```python
from build123d import *

# Parameters (mm, degrees)
F0_W     = 10
F0_H     = 10
F1_DEPTH = 10
F2_W     = 5
F2_H     = 5
F3_DEPTH = 5
F4_W     = 5
F4_H     = 5
F5_DEPTH = 5
F6_W     = 5
F6_H     = 5
F7_DEPTH = 5
F8_R     = 1.295802
F9_DEPTH = 25


with BuildPart() as f1:
    # F0 (on Top) → F1 (new body)
    with BuildSketch(Plane.XY):
        with Locations((-5, 5)):
            Rectangle(F0_W, F0_H)
    extrude(amount=F1_DEPTH)

    # F2 (on face) → F3 (join)
    with BuildSketch(Plane.YZ):
        with Locations((7.5, 2.5)):
            Rectangle(F2_W, F2_H)
    extrude(amount=F3_DEPTH)

    # F4 (on face) → F5 (join)
    with BuildSketch(Plane.XZ):
        with Locations((-7.5, 2.5)):
            Rectangle(F4_W, F4_H)
    extrude(amount=F5_DEPTH)

    # F6 (on face) → F7 (join)
    with BuildSketch(Plane.XY.offset(10)):
        with Locations((-7.5, 7.5)):
            Rectangle(F6_W, F6_H)
    extrude(amount=F7_DEPTH)

    # F8 (on face) → F9 (cut)
    with BuildSketch(Plane.XY.offset(15)):
        with Locations((-7.5, 7.526434)):
            Circle(F8_R)
    extrude(amount=-F9_DEPTH, mode=Mode.SUBTRACT)


solid = f1.part
```
Could you check a few things on this model? Use its own coordinates, in mm. A direction names the side the tool comes from. Round coordinates to 2 decimals unless told otherwise and drop trailing zeros. Loops run counter-clockwise (first coordinate to the right, second up) from the corner with the lowest first, then second, coordinate; pieces in that order, holes last. Notation, with made-up numbers: (7.5, 86) - (54.5, 86) arc R16 cw to (54.5, 97) - close; hole circle Ø11 at (36, -34.75). An arc over 180 degrees is marked (long way). Answer in a Markdown table with one row per item. Add a question column.
(1) If we section it at B-B (y = 8.5): Please give me the cut outline in (x, z), plus the area to 3 significant figures.
(2) I'm going to push flat-ended pins straight in: pin 1 (5.5 mm diameter, centred on x = 2, z = 2, fed in from -Y); pin 2 (4 mm diameter, centred on x = 3.5, y = 7.5, fed in from +Z); pin 3 (1.5 mm diameter, centred on x = -4, y = -2.5, fed in from -Z); pin 4 (2 mm diameter, centred on y = 1.5, z = 6, fed in from +X). Where does each tip first touch, or does it pass through?
(3) If we mould it in two halves opening along X, with no side actions, what happens to faces 1 (the face through (-10, 4, 6)), 2 (the face through (5, 7, 3)), 3 (the face through (-6.803, 8.619, 7.605)), 4 (the face through (-8, -2, 5))? For each: pulls with the +X half, pulls with the -X half, needs draft (parallel to the pull), parting line crosses it, or undercut.
(4) If we section it at D-D (x = -5.75): Please give me the cut outline in (y, z).
(5) I need wall thicknesses on line 1 along Y through (x, z) = (-7.5, 6.5); line 2 along X through (y, z) = (-2.25, 2.5); line 3 along X through (y, z) = (2.5, 4.5). Which ranges of each line are inside material? Lowest first, please.
(6) If we section it at A-A (x = -7.5): Please give me the cut outline in (y, z), plus the area to 3 significant figures.
(7) For faces 5 (the face through (-8, 5, 12)), 6 (the face through (2, 7, 5)), 7 (the face through (-8, -5, 3)), 8 (the face through (-5, -2, 2)), 9 (the face through (-4, 4, 0)), which set-ups out of +Z, -Z, +X, -X, +Y, -Y let a thin tool reach every point of the face, with its end or its side?
(8) If we section it at C-C (z = 7.25): Please give me the cut outline in (x, y), plus the area to 3 significant figures.
Model answer:
| question | item | result |
|---|---|---|
| 1 | outline | (-10, 0) - (-8.36, 0) - (-8.36, 15) - (-10, 15) - close; (-6.64, 0) - (5, 0) - (5, 5) - (0, 5) - (0, 10) - (-5, 10) - (-5, 15) - (-6.64, 15) - close |
| 1 | area | 124 mm² |
| 2 | pin 1 | stops at y = 0 |
| 2 | pin 2 | stops at z = 5 |
| 2 | pin 3 | passes through |
| 2 | pin 4 | stops at x = 0 |
| 3 | face 1 | pulls with the -X half |
| 3 | face 2 | pulls with the +X half |
| 3 | face 3 | undercut |
| 3 | face 4 | needs draft |
| 4 | outline | (-5, 0) - (10, 0) - (10, 15) - (5, 15) - (5, 10) - (0, 10) - (0, 5) - (-5, 5) - close |
| 5 | line 1 | y = 0 to 6.23, 8.82 to 10 |
| 5 | line 2 | x = -10 to -5 |
| 5 | line 3 | x = -10 to 0 |
| 6 | outline | (-5, 0) - (6.23, 0) - (6.23, 15) - (5, 15) - (5, 10) - (0, 10) - (0, 5) - (-5, 5) - close; (8.82, 0) - (10, 0) - (10, 15) - (8.82, 15) - close |
| 6 | area | 111 mm² |
| 7 | face 5 | +Z, +X, -X, -Y |
| 7 | face 6 | +Z, +X, +Y, -Y |
| 7 | face 7 | +Z, -Z, +X, -X, -Y |
| 7 | face 8 | +Z, -Z, +X, -Y |
| 7 | face 9 | -Z, +X, -X, +Y, -Y |
| 8 | outline | (-10, 0) - (0, 0) - (0, 10) - (-10, 10) - close; hole circle Ø2.59 at (-7.5, 7.53) |
| 8 | area | 94.7 mm² |
